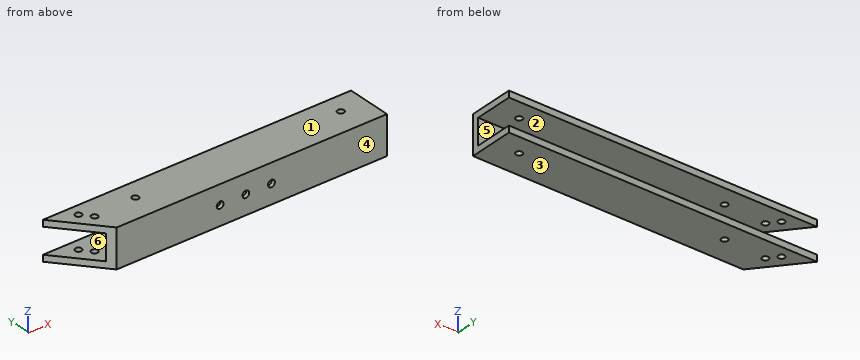
```python
from build123d import *

# Parameters (mm, degrees)
SKETCH1_W                                            = 304.8
SKETCH1_H                                            = 38.1
BOSS_EXTRUDE1_DEPTH                                  = 44.45
SKETCH2_W                                            = 304.8
SKETCH2_H                                            = 25.4
CUT_EXTRUDE1_DEPTH                                   = 38.1
CUT_EXTRUDE3_DEPTH                                   = 38.1
SKETCH5_R                                            = 3.175
CUT_EXTRUDE4_DEPTH                                   = 6.35
CSK_SLOT_FOR_1_4_FLAT_HEAD_MACHINE_SCREW_D           = 6.7564
CSK_SLOT_FOR_1_4_FLAT_HEAD_MACHINE_SCREW_CSINK_D     = 12.8778
CSK_SLOT_FOR_1_4_FLAT_HEAD_MACHINE_SCREW_CSINK_ANGLE = 100
SKETCH12_R                                           = 3.175
CUT_EXTRUDE5_DEPTH                                   = 6.35


with BuildPart() as part:
    # Sketch1 → Boss-Extrude1 (new body)
    with BuildSketch(Plane(origin=(0, 0, 0), x_dir=(1, 0, 0), z_dir=(0, 1, 0))):
        Rectangle(SKETCH1_W, SKETCH1_H)
    extrude(amount=BOSS_EXTRUDE1_DEPTH)

    # Sketch2 → Cut-Extrude1 (cut)
    with BuildSketch(Plane(origin=(0, 44.45, 0), x_dir=(1, 0, 0), z_dir=(0, 1, 0))):
        Rectangle(SKETCH2_W, SKETCH2_H)
    extrude(amount=-CUT_EXTRUDE1_DEPTH, mode=Mode.SUBTRACT)

    # Sketch4 → Cut-Extrude3 (cut)
    with BuildSketch(Plane.XY.offset(19.05)):
        Polygon((-152.4, 44.45), (-115.102021394, 0), (-152.4, 0), align=None)
    extrude(amount=-CUT_EXTRUDE3_DEPTH, mode=Mode.SUBTRACT)

    # Sketch5 → Cut-Extrude4 (cut)
    with BuildSketch(Plane.XY.offset(19.05)):
        with Locations((-126.344430286, 33.155873788)):
            Circle(SKETCH5_R)
        with Locations((-118.181027643, 23.42710936)):
            Circle(SKETCH5_R)
    cut_extrude4 = extrude(amount=-CUT_EXTRUDE4_DEPTH, mode=Mode.SUBTRACT)

    # Mirror1: Cut-Extrude4 across plane
    add(cut_extrude4.mirror(Plane.XY), mode=Mode.SUBTRACT)

    # CSK SLOT for 1/4 Flat Head Machine Screw (100)1 (through all)
    with Locations(Plane(origin=(0, 6.35, 0), x_dir=(1, 0, 0), z_dir=(0, 1, 0))):
        with Locations((-12.7, 0), (12.7, 0), (38.1, 0)):
            CounterSinkHole(CSK_SLOT_FOR_1_4_FLAT_HEAD_MACHINE_SCREW_D / 2, CSK_SLOT_FOR_1_4_FLAT_HEAD_MACHINE_SCREW_CSINK_D / 2, counter_sink_angle=CSK_SLOT_FOR_1_4_FLAT_HEAD_MACHINE_SCREW_CSINK_ANGLE)

    # Sketch12 → Cut-Extrude5 (cut)
    with BuildSketch(Plane.XY.offset(19.05)):
        with Locations((-76.2, 25.4)):
            Circle(SKETCH12_R)
        with Locations((127, 25.4)):
            Circle(SKETCH12_R)
    cut_extrude5 = extrude(amount=-CUT_EXTRUDE5_DEPTH, mode=Mode.SUBTRACT)

    # Mirror2: Cut-Extrude5 across plane
    add(cut_extrude5.mirror(Plane.XY), mode=Mode.SUBTRACT)


solid = part.part
```
Source: CAD feature listing. Evaluate the final solid. Frame: model axes, mm. Face numbers are marked on the shaded views. A direction names the side the tool comes from. Round coordinates to 2 decimals unless told otherwise and drop trailing zeros. Order: outer loops, then holes, each group sorted by start corner. A loop starts at its lowest first (then second) coordinate and runs counter-clockwise, first axis right, second up. Notation, with made-up numbers: (12.5, 72.5) -> (63.5, 72.5) arc R22 ccw to (63.5, 84.5) -> close; hole circle Ø1 at (-40, 80.25). An arc over 180 degrees is marked (long way). Use CSV: the item, a comma, the result in double quotes.
(1) Section B-B on x = 38.1. Return the cut outline in (y, z).
Report:
outline,"(0, -19.05) -> (44.45, -19.05) -> (44.45, -12.7) -> (6.35, -12.7) -> (6.35, -6.44) -> (3.78, -3.38) -> (0, -3.38) -> close; (0, 3.38) -> (3.78, 3.38) -> (6.35, 6.44) -> (6.35, 12.7) -> (44.45, 12.7) -> (44.45, 19.05) -> (0, 19.05) -> close"
(2) Access query for the marked faces 1 and 2. Directions: +Z, -Z, +X, -X, +Y, -Y. A direction counts if a zero-diameter tool reaches every point of the face in a straight line with its end or side. Return the directions, or none.
Report:
face 1,"+Z, +X, -X, +Y, -Y"
face 2,"+X, -X, +Y"
(3) Section A-A on z = 0. Return the cut outline in (x, y).
Report:
outline,"(-120.43, 6.35) -> (-115.1, 0) -> (-16.08, 0) -> (-16.08, 3.78) -> (-19.14, 6.35) -> close; (-9.32, 0) -> (9.32, 0) -> (9.32, 3.78) -> (6.26, 6.35) -> (-6.26, 6.35) -> (-9.32, 3.78) -> close; (16.08, 0) -> (34.72, 0) -> (34.72, 3.78) -> (31.66, 6.35) -> (19.14, 6.35) -> (16.08, 3.78) -> close; (41.48, 0) -> (152.4, 0) -> (152.4, 6.35) -> (44.54, 6.35) -> (41.48, 3.78) -> close"
(4) Ray query, L1, parallel to X at y = 4.5, z = 2.5; L2, parallel to Z at x = 65, y = 22; L3, parallel to Y at x = -76.2, z = -16.5 (3 decimals). Return the intervals inside material, ascending.
Report:
L1,"-118.88 to -16.12, -9.28 to 9.28, 16.12 to 34.68, 41.52 to 152.4"
L2,"-19.05 to -12.7, 12.7 to 19.05"
L3,"0 to 22.225, 28.575 to 44.45"
(5) Pull-direction query (Z, two-part tool) for the marked faces 3, 4, 5 and 6; classes: +Z half, -Z half, draft (parallel to the pull), parting line (faces both ways), or undercut.
Report:
face 3,"-Z half"
face 4,"draft"
face 5,"undercut"
face 6,"undercut"
(6) Section D-D on y = 17. Return the cut outline in (x, z), and give its area (3 significant figures).
Report:
outline,"(-129.37, -19.05) -> (152.4, -19.05) -> (152.4, -12.7) -> (-129.37, -12.7) -> close; (-129.37, 12.7) -> (152.4, 12.7) -> (152.4, 19.05) -> (-129.37, 19.05) -> close"
area,"3,580 mm^2"
(7) First-contact query: pin 1 Ø2 at (x, z) = (28, 2.5) entering from +Y; pin 2 Ø7.5 at (x, z) = (62, -2.5) entering from +Y; pin 3 Ø5 at (x, y) = (127, 25.4) entering from -Z; pin 4 Ø9 at (x, z) = (-12.7, 0) entering from +Y. Flat tips, straight axial feed; report the tip coordinate or a pass-through.
Report:
pin 1,"y = 6.35"
pin 2,"y = 6.35"
pin 3,"through"
pin 4,"y = 4.72"
(8) Section C-C on x = -76.2. Return the cut outline in (y, z) (3 decimals).
Report:
outline,"(0, -19.05) -> (22.225, -19.05) -> (22.225, -12.7) -> (6.35, -12.7) -> (6.35, 12.7) -> (22.225, 12.7) -> (22.225, 19.05) -> (0, 19.05) -> close; (28.575, -19.05) -> (44.45, -19.05) -> (44.45, -12.7) -> (28.575, -12.7) -> close; (28.575, 12.7) -> (44.45, 12.7) -> (44.45, 19.05) -> (28.575, 19.05) -> close"
